from build123d import *

# Parameters (mm, degrees)
SKETCH1_R           = 175
BOSS_EXTRUDE1_DEPTH = 1.6
SKETCH2_W           = 15
SKETCH2_H           = 100
CUT_EXTRUDE1_DEPTH  = 1.6
SKETCH3_W           = 60
SKETCH3_H           = 60
CUT_EXTRUDE2_DEPTH  = 2.6


with BuildPart() as part:
    # Sketch1 → Boss-Extrude1 (new body)
    with BuildSketch(Plane.XY):
        Circle(SKETCH1_R)
    extrude(amount=BOSS_EXTRUDE1_DEPTH)

    # Sketch2 → Cut-Extrude1 (cut)
    with BuildSketch(Plane.XY.offset(1.6)):
        with Locations((-120, 0)):
            Rectangle(SKETCH2_W, SKETCH2_H)
        with Locations((120, 0)):
            Rectangle(SKETCH2_W, SKETCH2_H)
    extrude(amount=-CUT_EXTRUDE1_DEPTH, mode=Mode.SUBTRACT)

    # Sketch3 → Cut-Extrude2 (cut, through all)
    with BuildSketch(Plane.XY.offset(1.6)):
        with Locations((0, -110)):
            Rectangle(SKETCH3_W, SKETCH3_H)
    extrude(amount=-CUT_EXTRUDE2_DEPTH, mode=Mode.SUBTRACT)


solid = part.part
Check sheet for the modelled part. Datum: model origin and axes. Units: mm. Give positions to 0.01 mm unless a question says otherwise; leave off trailing zeros. Write each loop counter-clockwise with the first axis right and the second up, starting at its lowest first coordinate (ties: lowest second). Pieces come first, ordered by that corner, then holes. Notation, with made-up numbers: M 27.5,36 L 48.5,36 A22 ccw 48.5,65 Z; hole C -2.5,87 d3. An arc over 180 degrees is marked long. Use one line per item in the form item = value.
(1) Section check A-A on y = 0. Record the boundary of the cut face in (x, z), plus the area to 3 significant figures.
Answer block:
outline = M -175,0 L -127.5,0 L -127.5,1.6 L -175,1.6 Z; M -112.5,0 L 112.5,0 L 112.5,1.6 L -112.5,1.6 Z; M 127.5,0 L 175,0 L 175,1.6 L 127.5,1.6 Z
area = 512 mm2
(2) Section check C-C on z = 0.3. Record the boundary of the cut face in (x, y).
Answer block:
outline = C 0,0 d350; hole M -127.5,-50 L -112.5,-50 L -112.5,50 L -127.5,50 Z; hole M -30,-140 L 30,-140 L 30,-80 L -30,-80 Z; hole M 112.5,-50 L 127.5,-50 L 127.5,50 L 112.5,50 Z
(3) Depth check by flat-ended pin: P1, Ø0.5, axis at x = 121, z = 1, coming from the -Y side; P2, Ø3, axis at x = 114, y = -71, coming from the -Z side; P3, Ø0.8, axis at y = -111, z = 1, coming from the +X side; P4, Ø0.5, axis at y = 16.5, z = 1, coming from the -X side. Enter the tip coordinate at first touch or a pass-through.
Answer block:
P1 = -126.67
P2 = 0
P3 = 135.62
P4 = -174.24
(4) Material ranges on line 1 along Y through (x, z) = (-4.5, 1.25); line 2 along X through (y, z) = (-89.5, 0.3); line 3 along X through (y, z) = (-90.5, 0.75), recorded low to high.
Answer block:
line_1 = -174.94 to -140, -80 to 174.94
line_2 = -150.38 to -30, 30 to 150.38
line_3 = -149.78 to -30, 30 to 149.78
(5) Section check B-B on x = 0. Record the boundary of the cut face in (y, z).
Answer block:
outline = M -175,0 L -140,0 L -140,1.6 L -175,1.6 Z; M -80,0 L 175,0 L 175,1.6 L -80,1.6 Z
(6) Section check D-D on x = -154. Record the boundary of the cut face in (y, z), plus the area to 3 significant figures.
Answer block:
outline = M -83.12,0 L 83.12,0 L 83.12,1.6 L -83.12,1.6 Z
area = 266 mm2
